Source: CAD feature listing. Evaluate the final solid. Frame: model axes, mm. A direction names the side the tool comes from. Give positions to 0.01 mm unless a question says otherwise; leave off trailing zeros. Order: outer loops, then holes, each group sorted by start corner. A loop starts at its lowest first (then second) coordinate and runs counter-clockwise, first axis right, second up. Notation, with made-up numbers: (-5.75, -30.75) -> (13.25, -30.75) arc R30 cw to (13.25, 6.25) -> close; hole circle Ø7 at (-2, 26.25). An arc over 180 degrees is marked (long way). Answer in a Markdown table with one row per item.
Autodesk Inventor part; units mm, degrees
ref_plane "Work Plane1" through (0, 25.4, -26.416) normal (-1, 0, 0) x (0, 0, 1)
ref_plane "YZ Plane" through (0, 0, 0) normal (1, 0, 0) x (0, 1, 0)
ref_plane "XZ Plane" through (0, 0, 0) normal (0, 1, 0) x (-1, 0, 0)
sketch "Sketch2" plane through (0, 0, 0) normal (0, 1, 0) x (-1, 0, 0)
  line L0 (-31.75, 31.75) -> (31.75, 31.75)
  line L1 (31.75, 31.75) -> (31.75, -31.75)
  line L2 (31.75, -31.75) -> (-31.75, -31.75)
  line L3 (-31.75, -31.75) -> (-31.75, 31.75)
  line L4 (-31.75, 31.75) -> (31.75, -31.75) construction
  line L5 (31.75, 31.75) -> (-31.75, -31.75) construction
  point P0 (0, 0)
  dimension "d3" = 63.5
  dimension "d4" = 63.5
extrude "Extrusion2" add sketch "Sketch2" along normal blind 25.4
fillet "Fillet1" radius 6.35 4 edges at (31.75, 12.7, 31.75) (31.75, 12.7, -31.75) (-31.75, 12.7, -31.75) (-31.75, 12.7, 31.75)
sketch "Sketch3" plane through (0, 25.4, 0) normal (0, 1, 0) x (1, 0, 0)
  arc A0 (-31.75, -25.4) -> (-25.4, -31.75) centre (-25.4, -25.4) ccw
  line L0 (-25.4, -31.75) -> (25.4, -31.75)
  arc A1 (25.4, -31.75) -> (31.75, -25.4) centre (25.4, -25.4) ccw
  line L1 (31.75, -25.4) -> (31.75, 25.4)
  arc A2 (31.75, 25.4) -> (25.4, 31.75) centre (25.4, 25.4) ccw
  line L2 (25.4, 31.75) -> (-25.4, 31.75)
  arc A3 (-25.4, 31.75) -> (-31.75, 25.4) centre (-25.4, 25.4) ccw
  line L3 (-31.75, 25.4) -> (-31.75, -25.4)
  line L4 (-26.416, 26.416) -> (26.416, 26.416)
  line L5 (26.416, 26.416) -> (26.416, -26.416)
  line L6 (26.416, -26.416) -> (-26.416, -26.416)
  line L7 (-26.416, -26.416) -> (-26.416, 26.416)
  point P0 (0, 0)
  dimension "d8" = 5.334
extrude "Extrusion3" cut sketch "Sketch3" against normal blind 20.066 contours L4 L5 L6 L7
ref_plane "Work Plane1" through (0, 25.4, -26.416) normal (-1, 0, 0) x (0, 0, 1)
fillet "Fillet2" radius 7.9375 4 edges at (-26.416, 15.367, 26.416) (-26.416, 15.367, -26.416) (26.416, 15.367, -26.416) (26.416, 15.367, 26.416)
sketch "Sketch6" plane through (-25.4, 0, 31.75) normal (0, 0, 1) x (1, 0, 0)
  line L0 (0, 0) -> (0, 25.4)
  line L1 (50.8, 0) -> (0, 0)
  line L2 (50.8, 25.4) -> (50.8, 0)
  line L3 (0, 25.4) -> (50.8, 25.4)
  circle A0 centre (25.4, 12.7) radius 1.27
  point P0 (25.4, 0)
  dimension "d31" = 2.54
  dimension "d32" = 12.7
  dimension "d33" = 25.4
hole "Hole3" at (0, 12.7, 31.75) direction (0, 0, -1) diameter 2.54 depth 76.2 tip angle 118
sketch "Sketch8" plane through (0, 0, 0) normal (0, -1, 0) x (1, 0, 0)
  point P0 (0, 0)
sketch "Sketch9" plane through (0, 0, 0) normal (0, -1, 0) x (1, 0, 0)
  line L0 (25.4, 28.575) -> (-15.875, 28.575)
  arc A0 (-15.875, 28.575) -> (-28.575, 15.875) centre (-15.875, 15.875) ccw
  line L1 (-28.575, 15.875) -> (-28.575, -15.875)
  arc A1 (-28.575, -15.875) -> (-15.875, -28.575) centre (-15.875, -15.875) ccw
  line L2 (-15.875, -28.575) -> (25.4, -28.575)
  arc A2 (25.4, -28.575) -> (28.575, -25.4) centre (25.4, -25.4) ccw
  line L3 (28.575, -25.4) -> (28.575, -1.27)
  line L4 (28.575, -1.27) -> (17.9256, -1.27)
  circle A3 centre (0, 0) radius 17.9705
  line L5 (17.9256, 1.27) -> (28.575, 1.27)
  line L6 (28.575, 1.27) -> (28.575, 25.4)
  arc A4 (28.575, 25.4) -> (25.4, 28.575) centre (25.4, 25.4) ccw
  circle A5 centre (-19.685, -19.685) radius 1.27
  circle A6 centre (-19.685, 19.685) radius 1.27
  dimension "d53" = 2.54
  dimension "d54" = 3.81
  dimension "d55" = 3.81
  dimension "d56" = 2.54
  dimension "d57" = 3.81
  dimension "d58" = 3.81
extrude "Extrusion6" cut sketch "Sketch9" against normal blind 25.4 contours A3 | A5 | A6
sketch "Sketch10" plane through (31.75, 0, 25.4) normal (1, 0, 0) x (0, 0, -1)
  circle A0 centre (25.4, 18.5) radius 3.175
  point P0 (25.4, 0)
  dimension "d61" = 6.35
extrude "Extrusion7" cut sketch "Sketch10" against normal blind 6.35
properties part number "basemotor"
(1) Section query C-C (x = 0). Return the cut outline in (y, z).
A:
| item | result |
|---|---|
| outline | (0, -31.75) -> (11.43, -31.75) -> (11.43, -26.42) -> (5.33, -26.42) -> (5.33, -17.97) -> (0, -17.97) -> close; (0, 17.97) -> (5.33, 17.97) -> (5.33, 26.42) -> (11.43, 26.42) -> (11.43, 31.75) -> (0, 31.75) -> close; (13.97, -31.75) -> (25.4, -31.75) -> (25.4, -26.42) -> (13.97, -26.42) -> close; (13.97, 26.42) -> (25.4, 26.42) -> (25.4, 31.75) -> (13.97, 31.75) -> close |
(2) Ray query, probe 1 along Z at (x, y) = (-14, 13.75); probe 2 along Z at (x, y) = (0, 2.2). Return the intervals inside material, ascending.
A:
| item | result |
|---|---|
| probe 1 | z = -31.75 to -26.42, 26.42 to 31.75 |
| probe 2 | z = -31.75 to -17.97, 17.97 to 31.75 |
(3) First-contact query: pin 1 Ø2 at (x, y) = (0, 12.7) entering from +Z; pin 2 Ø3.5 at (x, z) = (-19.685, 19.685) entering from +Y. Flat tips, straight axial feed; report the tip coordinate or a pass-through.
A:
| item | result |
|---|---|
| pin 1 | passes through |
| pin 2 | stops at y = 5.33 |
(4) Section query B-B (z = 0). Give the number of separate pieces and of enclosed holes in the cut face, plus the area to 3 significant figures.
A:
| item | result |
|---|---|
| separate pieces | 3 |
| enclosed holes | 0 |
| area | 327 mm^2 |
(5) Access query for faces 4 (the cylindrical face through (-24.15, 15.23, -24.03)), 5 (the cylindrical face through (29.12, 21.65, 0.41)), 6 (the cylindrical face through (-29.84, 12.88, -29.94)). Directions: +Z, -Z, +X, -X, +Y, -Y. A direction counts if a zero-diameter tool reaches every point of the face in a straight line with its end or side. Return the directions, or none.
A:
| item | result |
|---|---|
| face 4 | +Y |
| face 5 | +X |
| face 6 | -Z, -X, +Y, -Y |
(6) Pull-direction query (Y, two-part tool) for faces 1 (the flat face through (-26.416, 16, 0)), 2 (the cylindrical face through (-0.06, 13.97, 29.05)), 3 (the flat face through (-18, 5.334, -6)); classes: +Y half, -Y half, draft (parallel to the pull), parting line (faces both ways), or undercut.
A:
| item | result |
|---|---|
| face 1 | draft |
| face 2 | undercut |
| face 3 | +Y half |
